Geometry: see drawing. Coordinates: mm, zero at the bounding-box minimum. Give positions to 0.01 mm unless a question says otherwise; leave off trailing zeros. Loops run counter-clockwise (first coordinate to the right, second up) from the corner with the lowest first, then second, coordinate; pieces in that order, holes last. Notation, with made-up numbers: (-1.5, -34.75) - (23.5, -34.75) arc R23 ccw to (23.5, -2.75) - close; hole circle Ø1 at (29.25, 18). An arc over 180 degrees is marked (long way). Use one line per item in the form item = value.
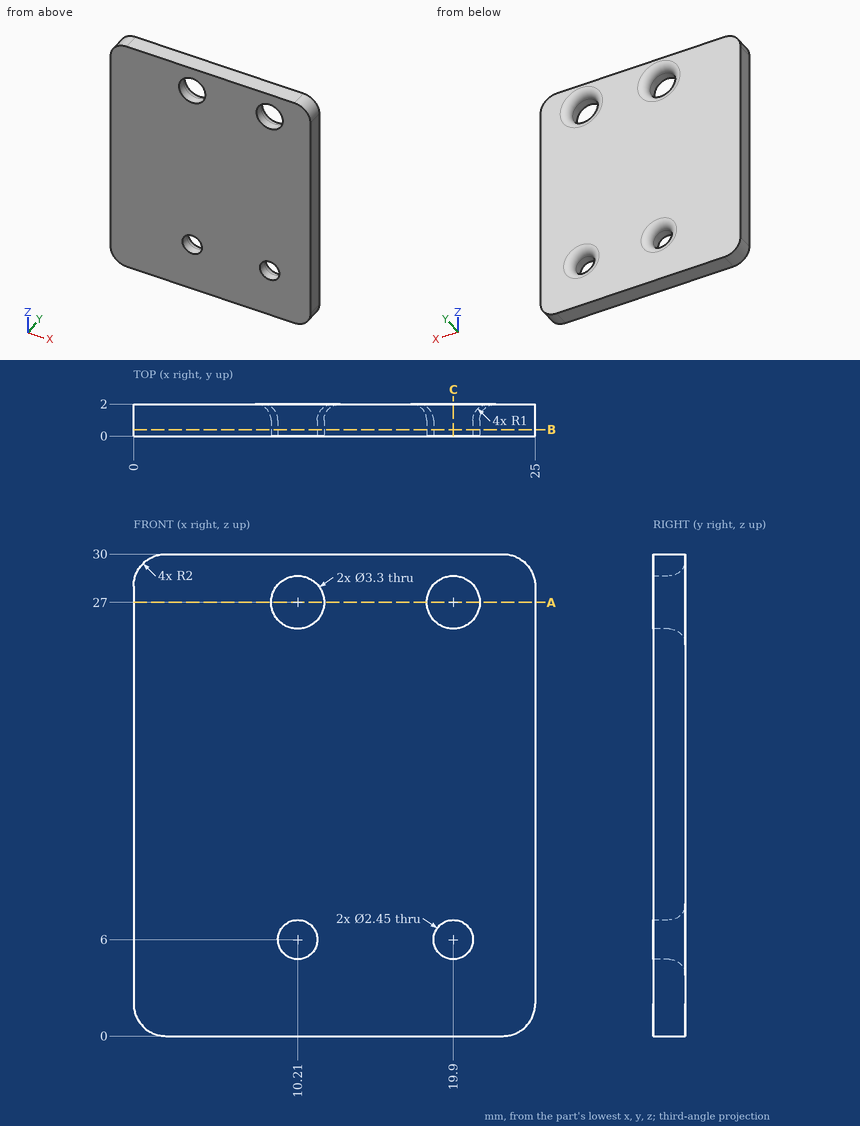
(1) Cut plane B-B (y = 0.4). Return the cut outline in (x, z) (3 decimals).
Solution:
outline = (0, 2) arc R2 ccw to (2, 0) - (23, 0) arc R2 ccw to (25, 2) - (25, 28) arc R2 ccw to (23, 30) - (2, 30) arc R2 ccw to (0, 28) - close; hole circle Ø3.3 at (10.21, 27); hole circle Ø2.45 at (10.21, 6); hole circle Ø3.3 at (19.9, 27); hole circle Ø2.45 at (19.9, 6)
(2) Cut plane C-C (x = 19.9). Return the cut outline in (y, z) (3 decimals), plus the area to 3 significant figures.
Solution:
outline = (0, 0) - (2, 0) - (2, 3.775) arc R1 ccw to (1, 4.775) - (0, 4.775) - close; (0, 7.225) - (1, 7.225) arc R1 ccw to (2, 8.225) - (2, 24.35) arc R1 ccw to (1, 25.35) - (0, 25.35) - close; (0, 28.65) - (1, 28.65) arc R1 ccw to (2, 29.65) - (2, 30) - (0, 30) - close
area = 47.6 mm2
(3) Material intervals for L1, parallel to X at y = 0.7, z = 27; L2, parallel to X at y = 0.7, z = 6 (3 decimals); L3, parallel to Z at x = 19.5, y = 1.2, sorted ascending. Write a range as from..to.
Solution:
L1 = 0..8.56, 11.86..18.25, 21.55..25
L2 = 0..8.985, 11.435..18.675, 21.125..25
L3 = 0..4.82, 7.18..25.38, 28.62..30
(4) Cut plane A-A (z = 27). Return the cut outline in (x, y).
Solution:
outline = (0, 0) - (8.56, 0) - (8.56, 1) arc R1 ccw to (7.56, 2) - (0, 2) - close; (11.86, 0) - (18.25, 0) - (18.25, 1) arc R1 ccw to (17.25, 2) - (12.86, 2) arc R1 ccw to (11.86, 1) - close; (21.55, 0) - (25, 0) - (25, 2) - (22.55, 2) arc R1 ccw to (21.55, 1) - close
(5) Pin query (flat end, axial travel): P1, Ø5.5, axis at x = 19.9, z = 27, coming from the +Y side. Return the tip coordinate at first contact, or that it passes through.
Solution:
P1 = 2
